Build history of the part. All positions in model axes, mm. Round coordinates to 2 decimals unless told otherwise and drop trailing zeros. One line per item, written item: value. Start each with the question number.
Item 1: Pin check, flat tips, straight feed: pin 1 (3 mm diameter, centred on x = 8, z = -350.5, fed in from -Y); pin 2 (11 mm diameter, centred on x = 0, z = 240, fed in from +Y); pin 3 (5.5 mm diameter, centred on x = 0, z = -240, fed in from +Y); pin 4 (10 mm diameter, centred on y = 19.5, z = 479, fed in from -X). Stop position of each tip, or through.
Item 2: Band-saw the part on A-A, the plane x = 0. Give the number of separate pieces and of enclosed holes in the cut face, then the cut area to 3 significant figures.
Item 3: Probe L1, parallel to X at y = 10, z = 400; L2, parallel to X at y = 20, z = 400; L3, parallel to X at y = 16.75, z = -263. List the from-to ranges inside material, lowest first.
```python
from build123d import *

# Parameters (mm, degrees)
BOSS_EXTRUDE1_DEPTH = 760
LPATTERN1_COUNT     = 2
LPATTERN1_PITCH     = 80
LPATTERN2_COUNT     = 9
LPATTERN2_PITCH     = 160


with BuildPart() as part:
    # Sketch1 → Boss-Extrude1 (new, symmetric)
    with BuildSketch(Plane.XY):
        with BuildLine():
            Line((-9.911771432, 13.106808119), (-11.43, 12.7))
            Line((-11.43, 12.7), (-14, 10.13))
            Line((-14, 10.13), (-14, 1.5))
            Line((-14, 1.5), (-12.5, 0))
            Line((-12.5, 0), (12.5, 0))
            Line((12.5, 0), (14, 1.5))
            Line((14, 1.5), (14, 10.13))
            Line((14, 10.13), (11.43, 12.7))
            Line((11.43, 12.7), (9.911771432, 13.106808119))
            ThreePointArc((9.911771432, 13.106808119), (9.10996999, 13.642554715), (8.8, 14.555696858))
            Line((8.8, 14.555696858), (8.8, 20.444303142))
            ThreePointArc((8.8, 20.444303142), (9.10996999, 21.357445285), (9.911771432, 21.893191881))
            Line((9.911771432, 21.893191881), (11.43, 22.3))
            Line((11.43, 22.3), (14, 24.87))
            Line((14, 24.87), (14, 26.5))
            ThreePointArc((14, 26.5), (13.416985894, 27.416985894), (12.5, 28))
            Line((12.5, 28), (-12.5, 28))
            ThreePointArc((-12.5, 28), (-13.416985894, 27.416985894), (-14, 26.5))
            Line((-14, 26.5), (-14, 24.87))
            Line((-14, 24.87), (-11.43, 22.3))
            Line((-11.43, 22.3), (-9.911771432, 21.893191881))
            ThreePointArc((-9.911771432, 21.893191881), (-9.10996999, 21.357445285), (-8.8, 20.444303142))
            Line((-8.8, 20.444303142), (-8.8, 14.555696858))
            ThreePointArc((-8.8, 14.555696858), (-9.10996999, 13.642554715), (-9.911771432, 13.106808119))
        make_face()
    extrude(amount=BOSS_EXTRUDE1_DEPTH, both=True)

    # Sketch2 → Cut-Revolve1 (revolve, cut)
    with BuildSketch(Plane(origin=(0, 0, 0), x_dir=(0, 0, -1), z_dir=(1, 0, 0)), mode=Mode.PRIVATE) as cut_revolve1_sk:
        Polygon((-720, 28), (-713, 28), (-713, 16), (-715.5, 16), (-715.5, 0), (-720, 0), align=None)
    cut_revolve1 = revolve(cut_revolve1_sk.sketch.rotate(Axis((0, 28, 720), (0, -1, 0)), 180), axis=Axis((0, 28, 720), (0, -1, 0)), mode=Mode.SUBTRACT)

    # LPattern1: Cut-Revolve1 ×2
    with Locations(*[(0, 0, -i * LPATTERN1_PITCH) for i in range(1, LPATTERN1_COUNT)]):
        add(cut_revolve1, mode=Mode.SUBTRACT)

    # Mirror1: Cut-Revolve1 across plane
    add(cut_revolve1.mirror(Plane.XY), mode=Mode.SUBTRACT)

    # Mirror1 copy 1 sketch → Mirror1 copy 1 (revolve, cut)
    with BuildSketch(Plane(origin=(0, 0, 80), x_dir=(0, 0, 1), z_dir=(1, 0, 0))):
        Polygon((-720, -28), (-713, -28), (-713, -16), (-715.5, -16), (-715.5, 0), (-720, 0), align=None)
    revolve(axis=Axis((0, 28, -640), (0, 1, 0)), mode=Mode.SUBTRACT)

    # LPattern2: Cut-Revolve1 ×9
    with Locations(*[(0, 0, -i * LPATTERN2_PITCH) for i in range(1, LPATTERN2_COUNT)]):
        add(cut_revolve1, mode=Mode.SUBTRACT)

    # LPattern2 copy 1 sketch → LPattern2 copy 1 (revolve, cut)
    with BuildSketch(Plane(origin=(0, 0, -240), x_dir=(0, 0, -1), z_dir=(1, 0, 0))):
        Polygon((-720, 28), (-713, 28), (-713, 16), (-715.5, 16), (-715.5, 0), (-720, 0), align=None)
    revolve(axis=Axis((0, 28, 480), (0, -1, 0)), mode=Mode.SUBTRACT)

    # LPattern2 copy 2 sketch → LPattern2 copy 2 (revolve, cut)
    with BuildSketch(Plane(origin=(0, 0, -400), x_dir=(0, 0, -1), z_dir=(1, 0, 0))):
        Polygon((-720, 28), (-713, 28), (-713, 16), (-715.5, 16), (-715.5, 0), (-720, 0), align=None)
    revolve(axis=Axis((0, 28, 320), (0, -1, 0)), mode=Mode.SUBTRACT)

    # LPattern2 copy 3 sketch → LPattern2 copy 3 (revolve, cut)
    with BuildSketch(Plane(origin=(0, 0, -560), x_dir=(0, 0, -1), z_dir=(1, 0, 0))):
        Polygon((-720, 28), (-713, 28), (-713, 16), (-715.5, 16), (-715.5, 0), (-720, 0), align=None)
    revolve(axis=Axis((0, 28, 160), (0, -1, 0)), mode=Mode.SUBTRACT)

    # LPattern2 copy 4 sketch → LPattern2 copy 4 (revolve, cut)
    with BuildSketch(Plane(origin=(0, 0, -720), x_dir=(0, 0, -1), z_dir=(1, 0, 0))):
        Polygon((-720, 28), (-713, 28), (-713, 16), (-715.5, 16), (-715.5, 0), (-720, 0), align=None)
    revolve(axis=Axis((0, 28, 0), (0, -1, 0)), mode=Mode.SUBTRACT)

    # LPattern2 copy 5 sketch → LPattern2 copy 5 (revolve, cut)
    with BuildSketch(Plane(origin=(0, 0, -880), x_dir=(0, 0, -1), z_dir=(1, 0, 0))):
        Polygon((-720, 28), (-713, 28), (-713, 16), (-715.5, 16), (-715.5, 0), (-720, 0), align=None)
    revolve(axis=Axis((0, 28, -160), (0, -1, 0)), mode=Mode.SUBTRACT)

    # LPattern2 copy 6 sketch → LPattern2 copy 6 (revolve, cut)
    with BuildSketch(Plane(origin=(0, 0, -1040), x_dir=(0, 0, -1), z_dir=(1, 0, 0))):
        Polygon((-720, 28), (-713, 28), (-713, 16), (-715.5, 16), (-715.5, 0), (-720, 0), align=None)
    revolve(axis=Axis((0, 28, -320), (0, -1, 0)), mode=Mode.SUBTRACT)

    # LPattern2 copy 7 sketch → LPattern2 copy 7 (revolve, cut)
    with BuildSketch(Plane(origin=(0, 0, -1200), x_dir=(0, 0, -1), z_dir=(1, 0, 0))):
        Polygon((-720, 28), (-713, 28), (-713, 16), (-715.5, 16), (-715.5, 0), (-720, 0), align=None)
    revolve(axis=Axis((0, 28, -480), (0, -1, 0)), mode=Mode.SUBTRACT)

    # LPattern2 copy 8 sketch → LPattern2 copy 8 (revolve, cut)
    with BuildSketch(Plane(origin=(0, 0, -1360), x_dir=(0, 0, -1), z_dir=(1, 0, 0))):
        Polygon((-720, 28), (-713, 28), (-713, 16), (-715.5, 16), (-715.5, 0), (-720, 0), align=None)
    revolve(axis=Axis((0, 28, -640), (0, -1, 0)), mode=Mode.SUBTRACT)


solid = part.part
```
Output:
1. pin 1: stops at y = 0
1. pin 2: stops at y = 16
1. pin 3: passes through
1. pin 4: stops at x = -13.63
2. separate pieces: 20
2. enclosed holes: 0
2. area: 36,600 mm²
3. L1: x = -14 to -4.5, 4.5 to 14
3. L2: x = -8.8 to -7, 7 to 8.8
3. L3: x = -8.8 to 8.8
